Could you check a few things on this model? Use its own coordinates, in mm. A direction names the side the tool comes from. Coordinates: 2 decimals unless noted, no trailing zeros. Order: outer loops, then holes, each group sorted by start corner. A loop starts at its lowest first (then second) coordinate and runs counter-clockwise, first axis right, second up. Notation, with made-up numbers: (-35.5, -38.75) -> (9.5, -38.75) arc R33 ccw to (9.5, -9.75) -> close; hole circle Ø2 at (22, -0.75). An arc over 180 degrees is marked (long way). Use a Markdown table: item, result. Add a question column.
1) If we section it at A-A (x = -16.64): Write out the boundary of the cut face in (y, z), plus the area to 3 significant figures.
2) If we section it at C-C (y = 13.5): Write out the boundary of the cut face in (x, z) (3 decimals).
3) If I drill on L1, parallel to X at y = 7.15, z = 0 (3 decimals); L2, parallel to Y at x = -36, z = 1 (3 decimals); L3, parallel to Y at x = -19, z = -3, over which ranges is the centre line in solid material (lowest first)? Write a range as [from, to].
4) If we section it at D-D (x = -9): Write out the boundary of the cut face in (y, z), plus the area to 3 significant figures.
5) Will these pins go through, and if not, where does the flat tip stop? pin 1 Ø0.7 at (x, z) = (-16.5, -7.5) entering from +Y; pin 2 Ø1 at (x, y) = (-17, -0.5) entering from +Z; pin 3 Ø11 at (x, z) = (-36.5, 2) entering from +Y (3 decimals).
6) If we section it at B-B (z = -4.75): Write out the boundary of the cut face in (x, y) (3 decimals).
7) Which directions (+Z, -Z, +X, -X, +Y, -Y) give clear straight access to the entire face, cutting with the end or side of a thin tool? Please do faces 4 (the cylindrical face through (0.329, 11.179, 1.044)), 5 (the cylindrical face through (1.479, -7.088, -1.928)), 6 (the flat face through (-38, 0, 11.43)), 7 (the flat face through (-9, 7.31, -2)).
8) Thinking about a two-plate mould opening in Z: for faces 1 (the flat face through (-14, 0, 9.98)), 2 (the flat face through (0, -6.86, 0)), 3 (the cylindrical face through (9.978, -0.096, 0.219)), which applies, +Z half, -Z half, draft (parallel to the pull), parting line (faces both ways), or undercut?
```python
from build123d import *

# Parameters (mm, degrees)
GEAR_BOX_DEPTH      = 6.86
GEAR_BOX_DEPTH_BACK = 6.86
MOTOR_DEPTH         = 5.715
MOTOR_DEPTH_BACK    = 5.715
SKETCH2_W           = 13.61
SKETCH2_H           = 22.86
SKETCH3_R           = 1.51
SKETCH3_R_2         = 3.645
SKETCH3_R_3         = 2.43
SPACER_DEPTH        = 0.45
SPACER_BACK_START   = 0.45
SKETCH5_R           = 3.645
SKETCH5_R_2         = 2.43
SPACER_BACK_DEPTH   = 0.45
SKETCH4_R           = 1.095
OUTPUT_SHAFT_DEPTH  = 8.76
SKETCH7_R           = 1.15
CUT_EXTRUDE1_DEPTH  = 5


with BuildPart() as part:
    # Sketch1 → Gear Box (new, two sides: drawn at the far end of the back side and taken through both)
    with BuildSketch(Plane(origin=(0, 0, 0), x_dir=(1, 0, 0), z_dir=(0, 1, 0)).offset(-GEAR_BOX_DEPTH_BACK)):
        with BuildLine():
            Line((0, 9.98), (-28.425, 9.98))
            Line((-28.425, 9.98), (-28.425, 12.395))
            Line((-28.425, 12.395), (-30.84, 12.395))
            Line((-30.84, 12.395), (-30.84, -12.395))
            Line((-30.84, -12.395), (-28.425, -12.395))
            Line((-28.425, -12.395), (-28.425, -9.98))
            Line((-28.425, -9.98), (0, -9.98))
            ThreePointArc((0, -9.98), (9.98, 0), (0, 9.98))
        make_face()
    extrude(amount=GEAR_BOX_DEPTH + GEAR_BOX_DEPTH_BACK)

    # Sketch2 → Motor (add, two sides: drawn at the far end of the back side and taken through both)
    with BuildSketch(Plane(origin=(0, 0, 0), x_dir=(1, 0, 0), z_dir=(0, 1, 0)).offset(-MOTOR_DEPTH_BACK)):
        with Locations((-37.645, 0)):
            Rectangle(SKETCH2_W, SKETCH2_H)
    extrude(amount=MOTOR_DEPTH + MOTOR_DEPTH_BACK)

    # Sketch3 → Spacer (add)
    # profile 1 of 2: a face of its own
    with BuildSketch(Plane(origin=(0, 6.86, 0), x_dir=(1, 0, 0), z_dir=(0, 1, 0))):
        with Locations(Location((-9, 1.6, 0), (0, 0, 270))):
            Circle(SKETCH3_R)
    # profile 2 of 2: a face of its own
    with BuildSketch(Plane(origin=(0, 6.86, 0), x_dir=(1, 0, 0), z_dir=(0, 1, 0))):
        with Locations(Location((0, 0, 0), (0, 0, 270))):
            Circle(SKETCH3_R_2)
        with Locations(Location((0, 0, 0), (0, 0, 270))):
            Circle(SKETCH3_R_3, mode=Mode.SUBTRACT)
    extrude(amount=SPACER_DEPTH)

    # Sketch5 → Spacer(back) (add)
    with BuildSketch(Plane.XZ.offset(6.86).offset(SPACER_BACK_START)):
        with Locations(Location((0, 0, 0), (0, 0, 90))):
            Circle(SKETCH5_R)
        with Locations(Location((0, 0, 0), (0, 0, 90))):
            Circle(SKETCH5_R_2, mode=Mode.SUBTRACT)
    extrude(amount=-SPACER_BACK_DEPTH)

    # Sketch4 → Output Shaft (add)
    with BuildSketch(Plane(origin=(0, 6.86, 0), x_dir=(1, 0, 0), z_dir=(0, 1, 0))):
        with Locations(Location((0, 0, 0), (0, 0, 270))):
            Circle(SKETCH4_R)
    extrude(amount=OUTPUT_SHAFT_DEPTH)

    # Sketch7 → Cut-Extrude1 (cut)
    with BuildSketch(Plane(origin=(0, 6.86, 0), x_dir=(1, 0, 0), z_dir=(0, 1, 0))):
        with Locations(Location((-16.64, 7.30523239, 0), (0, 0, 270))):
            Circle(SKETCH7_R)
        with Locations(Location((-16.64, -7.5, 0), (0, 0, 270))):
            Circle(SKETCH7_R)
    extrude(amount=-CUT_EXTRUDE1_DEPTH, mode=Mode.SUBTRACT)


solid = part.part
```
Answer sheet:
| question | item | result |
|---|---|---|
| 1 | outline | (-6.86, -9.98) -> (6.86, -9.98) -> (6.86, -8.46) -> (1.86, -8.46) -> (1.86, -6.16) -> (6.86, -6.16) -> (6.86, 6.35) -> (1.86, 6.35) -> (1.86, 8.65) -> (6.86, 8.65) -> (6.86, 9.98) -> (-6.86, 9.98) -> close |
| 1 | area | 251 mm2 |
| 2 | outline | circle Ø2.19 at (0, 0) |
| 3 | L1 | [-3.645, -2.43], [-1.095, 1.095], [2.43, 3.645] |
| 3 | L2 | [-5.715, 5.715] |
| 3 | L3 | [-6.86, 6.86] |
| 4 | outline | (-6.86, -9.98) -> (6.86, -9.98) -> (6.86, -3.11) -> (7.31, -3.11) -> (7.31, -0.09) -> (6.86, -0.09) -> (6.86, 9.98) -> (-6.86, 9.98) -> close |
| 4 | area | 275 mm2 |
| 5 | pin 1 | y = 1.86 |
| 5 | pin 2 | z = 9.98 |
| 5 | pin 3 | y = 5.715 |
| 6 | outline | (-44.45, -5.715) -> (-30.84, -5.715) -> (-30.84, -6.86) -> (8.777, -6.86) -> (8.777, 6.86) -> (-30.84, 6.86) -> (-30.84, 5.715) -> (-44.45, 5.715) -> close |
| 7 | face 4 | +Y |
| 7 | face 5 | -Y |
| 7 | face 6 | +Z, -X, +Y, -Y |
| 7 | face 7 | +Z, -Z, -X, +Y |
| 8 | face 1 | +Z half |
| 8 | face 2 | undercut |
| 8 | face 3 | parting line |
